The listing builds one solid part. Answer for the finished solid, in the listing's coordinates (mm). A direction names the side the tool comes from. Give positions to 0.01 mm unless a question says otherwise; leave off trailing zeros. Write each loop counter-clockwise with the first axis right and the second up, starting at its lowest first coordinate (ties: lowest second). Pieces come first, ordered by that corner, then holes. Notation, with made-up numbers: (53, 71) -> (82, 71) arc R16 cw to (82, 92) -> close; hole circle Ø5 at (-16, 53.25). An arc over 180 degrees is marked (long way). Put each result on its own line as item: value. Start each with the question number.
1) A cutting plane is placed at B-B (x = 20). Write down the section's boundary in (y, z), then the cut area to 3 significant figures.
2) For a pull along Z with two mould halves and no side action, classify faces 1 (the cylindrical face through (-5.708, 0.087, 0.388)), 2 (the cylindrical face through (3.338, -1.802, 5.723)), 3 (the flat face through (-8, 0, 0)) as released by +Z, released by -Z, zero draft, split by the parting line, or undercut.
3) Flat-ended cylindrical pins translate along their axes: pin 1 Ø5 at (x, z) = (12.5, -5.5) entering from +Y; pin 2 Ø1 at (x, z) = (8.5, -1) entering from +Y; pin 3 Ø8 at (x, y) = (19.5, -4) entering from -Z. Find the tip coordinate at first contact, or state that the pin passes through.
4) Find the intervals of material crossed by line 1 along X through (y, z) = (0, -2.75); line 2 along X through (y, z) = (6.5, -3.75); line 3 along Y through (x, z) = (-4, -4), in increasing order. Write a range as from..to.
5) For faces 4 (the cylindrical face through (10.958, 3.286, -4.285)), 5 (the flat face through (-2, 0, 8.5)), 6 (the cylindrical face through (26.146, -1.802, 5.723)), determine the directions among +Z, -Z, +X, -X, +Y, -Y from which every point of the face is accessible in a straight line to the end or side of a thin tool.
6) A cutting plane is placed at A-A (x = -4). Write down the section's boundary in (y, z), then the cut area to 3 significant figures.
from build123d import *

# Parameters (mm, degrees)
EXTRUDE_1_DEPTH     = 8
SKETCH_3_OUTSIDE_W  = 198.604
SKETCH_3_OUTSIDE_H  = 201.234
SKETCH_3_OUTSIDE_R  = 8
CUT_EXTRUDE_1_DEPTH = 48.797315127
CUT_EXTRUDE_1_DRAFT = -60
FILLET_1_R          = 0.6
SKETCH_4_R          = 1.6
CUT_EXTRUDE_2_DEPTH = 43.770706486
SKETCH_5_R          = 1.75
CUT_EXTRUDE_3_DEPTH = 44.607147732


with BuildPart() as part:
    # Эскиз1 → Повернуть1 (revolve)
    with BuildSketch(Plane.XY, mode=Mode.PRIVATE) as revolve_1_sk:
        with BuildLine():
            Line((0, 0), (0, 6))
            Line((0, 6), (6, 6))
            Line((6, 6), (6.307106781, 5.692893219))
            ThreePointArc((6.307106781, 5.692893219), (6.63153013, 5.476120467), (7.014213562, 5.4))
            Line((7.014213562, 5.4), (14.792893219, 5.4))
            ThreePointArc((14.792893219, 5.4), (14.984234935, 5.438060234), (15.146446609, 5.546446609))
            Line((15.146446609, 5.546446609), (15.6, 6))
            Line((15.6, 6), (36.4, 6))
            Line((36.4, 6), (38, 4.4))
            Line((38, 4.4), (38, 0))
            Line((38, 0), (0, 0))
        make_face()
    revolve(revolve_1_sk.sketch.rotate(Axis((0, 0, 0), (1, 0, 0)), 90), axis=Axis((0, 0, 0), (1, 0, 0)))

    # Эскиз2 → Бобышка-Вытянуть1 (add)
    with BuildSketch(Plane.ZY):
        Polygon((0, -9.814954576), (8.5, -4.907477288), (8.5, 4.907477288), (0, 9.814954576), (-8.5, 4.907477288), (-8.5, -4.907477288), align=None)
    extrude(amount=EXTRUDE_1_DEPTH)


with BuildPart() as cut_extrude_1_tool:
    # Эскиз3 outside → Вырез-Вытянуть1 (with draft: the straight prism first)
    with BuildSketch(Plane.ZY.offset(8)):
        Rectangle(SKETCH_3_OUTSIDE_W, SKETCH_3_OUTSIDE_H)
        Circle(SKETCH_3_OUTSIDE_R, mode=Mode.SUBTRACT)
    extrude(amount=-CUT_EXTRUDE_1_DEPTH)
    # Вырез-Вытянуть1: the draft: its side faces are tilted about the plane it starts from
    cut_extrude_1_sides = [cut_extrude_1_tool.faces().sort_by_distance(p)[0] for p in [
        (16.398657563, -100.617, 0),
        (16.398657563, 0, 99.302),
        (16.398657563, 100.617, 0),
        (16.398657563, 0, -99.302),
        (16.398657563, 0, -8),
    ]]
    draft(cut_extrude_1_sides, Plane.ZY.offset(8), CUT_EXTRUDE_1_DRAFT)


with BuildPart() as part_1:
    add(part.part)

    # Вырез-Вытянуть1: cut by cut_extrude_1_tool
    add(cut_extrude_1_tool.part, mode=Mode.SUBTRACT)

    # Скругление1
    fillet_1_edges = [part_1.edges().sort_by_distance(p)[0] for p in [
        (0, 0, -6),
    ]]
    fillet(fillet_1_edges, radius=FILLET_1_R)

    # Эскиз4 → Вырез-Вытянуть2 (cut, through all)
    with BuildSketch(Plane.XY.offset(8.5)):
        with Locations((-4, 0)):
            Circle(SKETCH_4_R)
    extrude(amount=-CUT_EXTRUDE_2_DEPTH, mode=Mode.SUBTRACT)

    # Эскиз5 → Вырез-Вытянуть3 (cut, through all)
    with BuildSketch(Plane(origin=(0, -7.361215932, 4.25), x_dir=(1, 0, 0), z_dir=(0, -0.8660254037844384, 0.5000000000000003))):
        with Locations(Location((-4, 0, 0), (0, 0, 270))):
            Circle(SKETCH_5_R)
    extrude(amount=-CUT_EXTRUDE_3_DEPTH, mode=Mode.SUBTRACT)


solid = part_1.part
Reply:
1. outline: circle Ø12 at (0, 0)
1. area: 113 mm2
2. face 1: undercut
2. face 2: split by the parting line
2. face 3: zero draft
3. pin 1: stops at y = 4.49
3. pin 2: stops at y = 5.38
3. pin 3: stops at z = -6
4. line 1: x = -8..-5.6, -2.4..38
4. line 2: x = -8..-5.75, -2.25..0
4. line 3: y = -7.51..-1.6, 1.6..3.43
5. face 4: none
5. face 5: +Z, +X, -X, +Y, -Y
5. face 6: +X
6. outline: (-9.81, 0) -> (-4.91, -8.5) -> (-1.6, -8.5) -> (-1.6, -1.1) -> (-8.24, 2.73) -> close; (-6.49, 5.77) -> (-1.6, 2.94) -> (-1.6, 8.5) -> (-4.91, 8.5) -> close; (1.6, -8.5) -> (4.91, -8.5) -> (6.49, -5.77) -> (1.6, -2.94) -> close; (1.6, 1.1) -> (8.24, -2.73) -> (9.81, 0) -> (4.91, 8.5) -> (1.6, 8.5) -> close
6. area: 149 mm2
